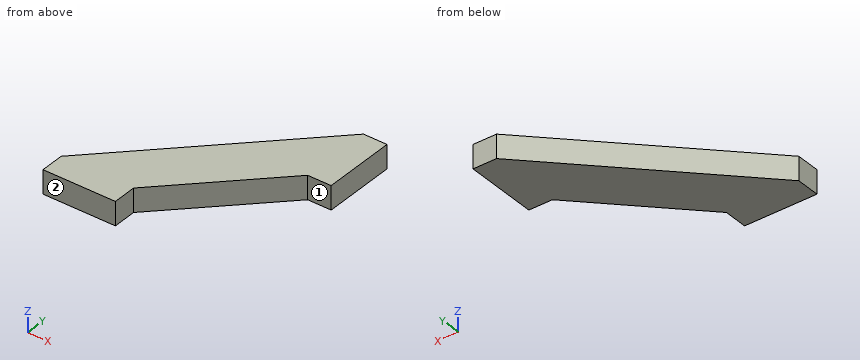
from build123d import *

# Parameters (mm, degrees)
F1_DEPTH = 12.3952
F2_W     = 38.1
F2_H     = 12.3952
F3_DEPTH = 12.3952
F4_W     = 38.1
F4_H     = 12.3952
F5_DEPTH = 12.3952


with BuildPart() as f1:
    # F0 (on Top) → F1 (new body)
    with BuildSketch(Plane.XY):
        Polygon((89.802561, 89.802561), (0, 0), (38.1, 0), (89.802561, 51.702561), align=None)
    extrude(amount=F1_DEPTH)

    # F2 (on face) → F3 (join)
    with BuildSketch(Plane.YZ.offset(89.802561)):
        with Locations((70.752561, 6.1976)):
            Rectangle(F2_W, F2_H)
    extrude(amount=F3_DEPTH)

    # F4 (on face) → F5 (join)
    with BuildSketch(Plane.XZ):
        with Locations((19.05, 6.1976)):
            Rectangle(F4_W, F4_H)
    extrude(amount=F5_DEPTH)


solid = f1.part
Model file for the job. Use its own axes, mm. Face numbers are marked on the shaded views. A direction names the side the tool comes from. Coordinates: 2 decimals unless noted, no trailing zeros. Write each loop counter-clockwise with the first axis right and the second up, starting at its lowest first coordinate (ties: lowest second). Pieces come first, ordered by that corner, then holes. Notation, with made-up numbers: (27, 61.5) - (86, 61.5) arc R29 cw to (86, 90.5) - close; hole circle Ø3 at (15, 66). An arc over 180 degrees is marked (long way). Write each question's results on one line, items separated by ' | '. Start each with the question number.
1) Cut at C-C (x = 25). Write the cut outline in (y, z), then the cut area to 3 significant figures.
2) Probe line 1 along Y through (x, z) = (98, 4.75); line 2 along X through (y, z) = (-2.5, 10); line 3 along X through (y, z) = (70.5, 9.75). List the from-to ranges inside material, lowest first. Write a range as from..to.
3) 3-axis set-ups, long thin cutter, end or side, ignore diameter. For the marked faces 1 and 2: which of +Z, -Z, +X, -X, +Y, -Y reach the whole face in a straight line?
4) Flat gauge pins, fed straight in: P1, Ø1.5, axis at x = 76.5, z = 2, coming from the +Y side; P2, Ø1, axis at y = 39, z = 4.5, coming from the -X side; P3, Ø3.5, axis at y = -5, z = 8.5, coming from the +X side. Where does each tip first touch, or does it go through?
5) Cut at B-B (y = 58). Write the cut outline in (x, z), then the cut area to 3 significant figures.
6) Cut at A-A (z = 7.25). Write the cut outline in (x, y).
Returned:
1) outline: (-12.4, 0) - (25, 0) - (25, 12.4) - (-12.4, 12.4) - close | area: 464 mm^2
2) line 1: 51.7..89.8 | line 2: 0..38.1 | line 3: 70.5..102.2
3) face 1: +Z, -Z, +X, -Y | face 2: +Z, -Z, +X, -X, -Y
4) P1: y = 77.25 | P2: x = 38.5 | P3: x = 38.1
5) outline: (58, 0) - (102.2, 0) - (102.2, 12.4) - (58, 12.4) - close | area: 548 mm^2
6) outline: (0, -12.4) - (38.1, -12.4) - (38.1, 0) - (89.8, 51.7) - (102.2, 51.7) - (102.2, 89.8) - (89.8, 89.8) - (0, 0) - close
